CAD build for the part. Positions are in the model's coordinates, mm. A direction names the side the tool comes from. Coordinates: 2 decimals unless noted, no trailing zeros. Loops run counter-clockwise (first coordinate to the right, second up) from the corner with the lowest first, then second, coordinate; pieces in that order, holes last. Notation, with made-up numbers: (-30.5, -37.75) -> (-16.5, -37.75) arc R27 ccw to (-16.5, -16.75) -> close; hole circle Ø2 at (27, 29.5). An arc over 180 degrees is marked (long way). Return JSON: item names as keys, results as strings. Group by question number.
(1) Tool access for faces 1 (the face through (-15, 0.2, 9)), 2 (the face through (-14.985, 3.455, -0.66)): list every direction of +Z, -Z, +X, -X, +Y, -Y with a clear straight run to the whole face (end or side of a thin tool).
(2) Probe L1, parallel to Z at x = 0, y = 5.5; L2, parallel to Z at x = 0, y = 0.15. List the from-to ranges inside material, lowest first.
(3) Flat gauge pins, fed straight in: pin 1 Ø1 at (y, z) = (2, 5) entering from -X; pin 2 Ø4 at (y, z) = (1.5, 10.5) entering from -X; pin 3 Ø18 at (x, z) = (0, 0) entering from -Y; pin 4 Ø2 at (y, z) = (3.5, -15) entering from +X. Where does each tip first touch, or does it go through?
(4) Saw through at C-C on y = 2.5. Write the cut outline in (x, z).
(5) Mould opens along Z. For faces 3 (the face through (-15, 6.8, -9)), 4 (the face through (15, 0, 5)), 5 (the face through (20.03, 3.46, -6.31)) say: pulls with the +Z half, pulls with the -Z half, needs draft (parallel to the pull), parting line crosses it, or undercut.
```python
from build123d import *

# Parameters (mm, degrees)
SKETCH1_R           = 21
SKETCH1_R_2         = 15
BOSS_EXTRUDE1_DEPTH = 7
SKETCH2_R           = 19.5
SKETCH2_R_2         = 16.5
CUT_EXTRUDE1_DEPTH  = 0.2
CHAMFER1_SIZE       = 0.3
SKETCH3_R           = 19.5
SKETCH3_R_2         = 16.5
CUT_EXTRUDE2_DEPTH  = 0.2


with BuildPart() as part:
    # Sketch1 → Boss-Extrude1 (new body)
    with BuildSketch(Plane(origin=(0, 0, 0), x_dir=(1, 0, 0), z_dir=(0, 1, 0))):
        Circle(SKETCH1_R)
        Circle(SKETCH1_R_2, mode=Mode.SUBTRACT)
    extrude(amount=BOSS_EXTRUDE1_DEPTH)

    # Sketch2 → Cut-Extrude1 (cut)
    with BuildSketch(Plane(origin=(0, 7, 0), x_dir=(1, 0, 0), z_dir=(0, 1, 0))):
        Circle(SKETCH2_R)
        Circle(SKETCH2_R_2, mode=Mode.SUBTRACT)
    extrude(amount=-CUT_EXTRUDE1_DEPTH, mode=Mode.SUBTRACT)

    # Chamfer1
    chamfer1_edges = [part.edges().sort_by_distance(p)[0] for p in [
        (-21, 0, 0),
        (-21, 7, 0),
        (-15, 0, 0),
        (-15, 7, 0),
    ]]
    chamfer(chamfer1_edges, length=CHAMFER1_SIZE)

    # Sketch3 → Cut-Extrude2 (cut)
    with BuildSketch(Plane.XZ):
        Circle(SKETCH3_R)
        Circle(SKETCH3_R_2, mode=Mode.SUBTRACT)
    extrude(amount=-CUT_EXTRUDE2_DEPTH, mode=Mode.SUBTRACT)


solid = part.part
```
Geometry results:
{
 "1": {"face 1": "-Y", "face 2": "+Y, -Y"},
 "2": {"L1": "-21 to -15, 15 to 21", "L2": "-20.85 to -19.5, -16.5 to -15.15, 15.15 to 16.5, 19.5 to 20.85"},
 "3": {"pin 1": "x = -20.51", "pin 2": "x = -19.2", "pin 3": "through", "pin 4": "x = 15.65"},
 "4": {"outline": "circle Ø42 at (0, 0); hole circle Ø30 at (0, 0)"},
 "5": {"face 3": "undercut", "face 4": "needs draft", "face 5": "parting line crosses it"}
}
